Input: part model. Units: mm. Frame: model coordinates. A direction names the side the tool comes from. Round coordinates to 2 decimals unless told otherwise and drop trailing zeros. Write each loop counter-clockwise with the first axis right and the second up, starting at its lowest first coordinate (ties: lowest second). Pieces come first, ordered by that corner, then holes. Notation, with made-up numbers: M -4.75,40 L 5.25,40 A29 ccw 5.25,69 Z; hole C 51,86.25 d3. An arc over 180 degrees is marked long. Use one line per item in the form item = value. Start each with the question number.
Autodesk Inventor part; units mm, degrees
ref_plane "YZ Plane" through (0, 0, 0) normal (1, 0, 0) x (0, 1, 0)
ref_plane "XZ Plane" through (0, 0, 0) normal (0, 1, 0) x (-1, 0, 0)
ref_plane "XY Plane" through (0, 0, 0) normal (0, 0, 1) x (1, 0, 0)
sketch "Sketch1" plane through (0, 0, 0) normal (0, 0, 1) x (1, 0, 0)
  line L0 (0, 0) -> (920, 0)
  line L1 (920, 0) -> (920, 30)
  line L2 (920, 30) -> (0, 30)
  line L3 (0, 30) -> (0, 0)
  dimension "d0" = 30
  dimension "d1" = 920
extrude "Extrusion1" add sketch "Sketch1" along normal blind 30
sketch "Sketch2" plane through (0, 30, 0) normal (0, 1, 0) x (1, 0, 0)
  line L0 (920, -30) -> (0, -30)
  line L1 (50, -30) -> (65, -30)
  line L2 (65, -30) -> (65, -15)
  line L3 (65, -15) -> (50, -15)
  line L4 (50, -15) -> (50, -30)
  line L5 (0, 0) -> (0, -30)
  line L6 (870, -30) -> (855, -30)
  line L7 (855, -30) -> (855, -15)
  line L8 (855, -15) -> (870, -15)
  line L9 (870, -15) -> (870, -30)
  line L10 (920, 0) -> (920, -30)
  dimension "d4" = 15
  dimension "d5" = 15
  dimension "d6" = 50
  dimension "d7" = 15
  dimension "d8" = 15
  dimension "d9" = 50
extrude "Extrusion2" add sketch "Sketch2" along normal blind 1120
sketch "Sketch3" plane through (0, 30, 0) normal (0, 1, 0) x (1, 0, 0)
  line L0 (920, 0) -> (0, 0)
  line L1 (855, -30) -> (65, -30)
  line L2 (430, 0) -> (460, 0)
  line L3 (460, 0) -> (460, -30)
  line L4 (460, -30) -> (430, -30)
  line L5 (430, -30) -> (430, 0)
  line L6 (920, 0) -> (920, -30)
  point P0 (460, -15)
  dimension "d12" = 30
  dimension "d13" = 460
extrude "Extrusion3" add sketch "Sketch3" along normal blind 1120
properties part number "Nhom30"
Item 1: First-contact query: pin 1 (4.5 mm diameter, centred on y = 660, z = 21.5, fed in from -X); pin 2 (7.5 mm diameter, centred on x = 866, y = 852.5, fed in from -Z); pin 3 (1 mm diameter, centred on y = 959, z = 25.5, fed in from +X). Flat tips, straight axial feed; report the tip coordinate or a pass-through.
Item 2: Ray query, line 1 (X direction, y = 1001.5, z = 23.75); line 2 (X direction, y = 392.5, z = 8); line 3 (Y direction, x = 618.5, z = 15.5). Return the intervals inside material, ascending. Write a range as from..to.
Item 3: Cut plane A-A (y = 1076). Output: boundary loops of the cut face in (x, z).
Item 4: Draft query along X for faces 3 (the face through (430, 582, 15)), 4 (the face through (218, 30, 15)), 5 (the face through (920, 15, 15)), 6 (the face through (458, 322, 0)). Return one class per face: +X half, -X half, draft (parallel to the pull), parting line (faces both ways), or undercut.
Item 5: Reachability of faces 1 (the face through (460, 582, 15)), 2 (the face through (458, 407, 30)) from +Z, -Z, +X, -X, +Y, -Y: full face, straight path, thin tool, end or side. Return the list, or none.
Item 6: Cut plane C-C (x = 108.5). Output: boundary loops of the cut face in (y, z), plus the area to 3 significant figures.
Item 7: Cut plane B-B (z = 9). Output: boundary loops of the cut face in (x, y), plus the area to 3 significant figures.
Final values:
q1.pin_1 = 50
q1.pin_2 = 15
q1.pin_3 = 870
q2.line_1 = 50..65, 430..460, 855..870
q2.line_2 = 430..460
q2.line_3 = 0..30
q3.outline = M 50,15 L 65,15 L 65,30 L 50,30 Z; M 430,0 L 460,0 L 460,30 L 430,30 Z; M 855,15 L 870,15 L 870,30 L 855,30 Z
q4.face_3 = undercut
q4.face_4 = undercut
q4.face_5 = +X half
q4.face_6 = draft
q5.face_1 = +Z, -Z, +Y
q5.face_2 = +Z, +X, -X, +Y, -Y
q6.outline = M 0,0 L 30,0 L 30,30 L 0,30 Z
q6.area = 900 mm^2
q7.outline = M 0,0 L 920,0 L 920,30 L 460,30 L 460,1150 L 430,1150 L 430,30 L 0,30 Z
q7.area = 61,200 mm^2
